Here's the drawing with two shaded views (mm, measured from the low corner). I have some questions. Round coordinates to 2 decimals unless told otherwise and drop trailing zeros. Order: outer loops, then holes, each group sorted by start corner. A loop starts at its lowest first (then second) coordinate and runs counter-clockwise, first axis right, second up. Notation, with made-up numbers: (-23, 66.25) - (20, 66.25) arc R26 cw to (20, 97.25) - close; hole circle Ø10 at (57.25, 13.25). An arc over 180 degrees is marked (long way). Return JSON: item names as keys, results as strings. Group by question number.
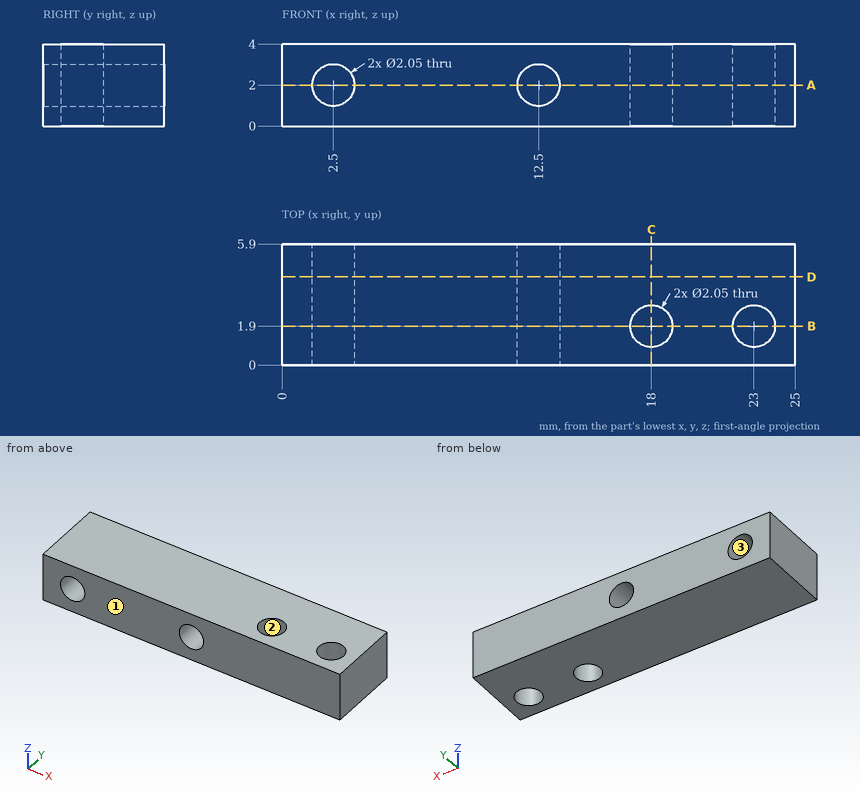
1) I want a section at D-D, the plane y = 4.3. List the corners of the cut face in (x, z) for me (3 decimals).
2) I want a section at A-A, the plane z = 2. List the corners of the cut face in (x, y) for me (3 decimals), plus the area to 3 significant figures.
3) If I drill on line 1 along X through (y, z) = (4.55, 2) (3 decimals); line 2 along Y through (x, z) = (18, 2.4) (3 decimals); line 3 along Z through (x, y) = (2.5, 1.85) (3 decimals), over which ranges is the centre line in solid material (lowest first)? Write a range as from..to.
4) We'd pull the mould along Y, two halves only. Please class the marked faces 1, 2 and 3: +Y half, -Y half, draft (parallel to the pull), parting line (faces both ways), or undercut.
5) I want a section at B-B, the plane y = 1.9. List the corners of the cut face in (x, z) for me (3 decimals).
6) I want a section at C-C, the plane x = 18. List the corners of the cut face in (y, z) for me (3 decimals), plus the area to 3 significant figures.
Outcome:
{
 "1": {"outline": "(0, 0) - (25, 0) - (25, 4) - (0, 4) - close; hole circle Ø2.05 at (2.5, 2); hole circle Ø2.05 at (12.5, 2)"},
 "2": {"outline": "(0, 0) - (1.475, 0) - (1.475, 5.9) - (0, 5.9) - close; (3.525, 0) - (11.475, 0) - (11.475, 5.9) - (3.525, 5.9) - close; (13.525, 0) - (25, 0) - (25, 5.9) - (13.525, 5.9) - close; hole circle Ø2.05 at (18, 1.9); hole circle Ø2.05 at (23, 1.9)", "area": "117 mm^2"},
 "3": {"line 1": "0..1.475, 3.525..11.475, 13.525..25", "line 2": "0..0.875, 2.925..5.9", "line 3": "0..0.975, 3.025..4"},
 "4": {"face 1": "-Y half", "face 2": "undercut", "face 3": "draft"},
 "5": {"outline": "(0, 0) - (16.975, 0) - (16.975, 4) - (0, 4) - close; (19.025, 0) - (21.975, 0) - (21.975, 4) - (19.025, 4) - close; (24.025, 0) - (25, 0) - (25, 4) - (24.025, 4) - close; hole circle Ø2.05 at (2.5, 2); hole circle Ø2.05 at (12.5, 2)"},
 "6": {"outline": "(0, 0) - (0.875, 0) - (0.875, 4) - (0, 4) - close; (2.925, 0) - (5.9, 0) - (5.9, 4) - (2.925, 4) - close", "area": "15.4 mm^2"}
}
